Design review of the part shown in the three views and the two pictorial views. Dimensions are in mm from the part's minimum x, y and z. Round coordinates to 2 decimals unless told otherwise and drop trailing zeros. Loops run counter-clockwise (first coordinate to the right, second up) from the corner with the lowest first, then second, coordinate; pieces in that order, holes last. Notation, with made-up numbers: M -26.5,27.5 L -15.5,27.5 A19 ccw -15.5,31.5 Z; hole C 77,-11 d5. An arc over 180 degrees is marked long. One line per question, with ' | ' between items. Start each with the question number.
1) We need section A-A (x = 3.9). Give the boundary of the cut face in (y, z).
2) We need section B-B (z = 3). Give the boundary of the cut face in (x, y).
3) We need section C-C (y = 0.5). Give the boundary of the cut face in (x, z).
4) We need section D-D (x = 7). Give the boundary of the cut face in (y, z), and give its area (3 significant figures).
5) For probe 1 along X at (y, z) = (7.75, 17); probe 2 along X at (y, z) = (5, 29.5); probe 3 along Y at (x, z) = (0.75, 26), list the stretches that pass through material, from the lowest coordinate up. Write a range as from..to.
6) For pin 1 Ø4 at (x, z) = (5.5, 32) entering from +Y; pin 2 Ø0.6 at (y, z) = (8, 9.5) entering from -X, all flat-tipped, find the tip position at first contact; note any pin that passes through.
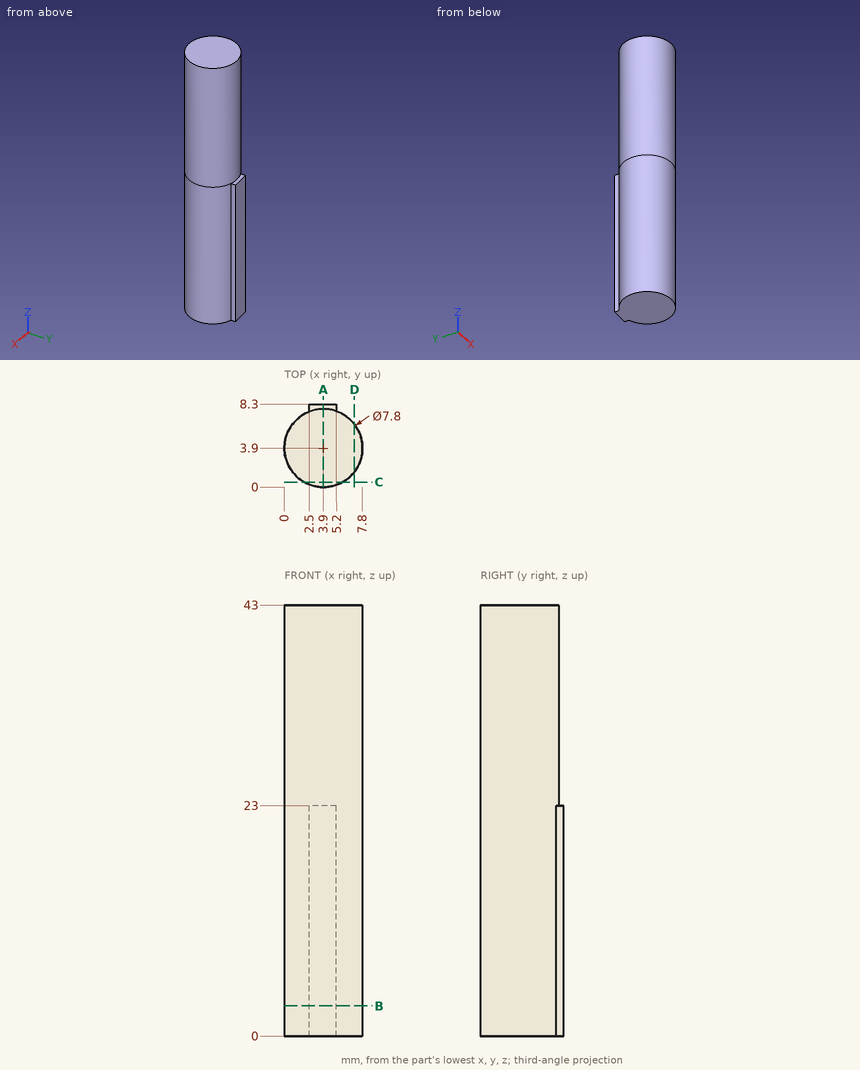
Answers below:
1) outline: M 0,0 L 8.3,0 L 8.3,23 L 7.8,23 L 7.8,43 L 0,43 Z
2) outline: M 2.5,7.54 A3.9 ccw long 5.2,7.58 L 5.2,8.3 L 2.5,8.3 Z
3) outline: M 1.99,0 L 5.81,0 L 5.81,43 L 1.99,43 Z
4) outline: M 1.53,0 L 6.27,0 L 6.27,43 L 1.53,43 Z | area: 204 mm^2
5) probe 1: 2.5..5.2 | probe 2: 0.16..7.64 | probe 3: 1.6..6.2
6) pin 1: y = 7.8 | pin 2: x = 2.5
